from build123d import *

# Parameters (mm, degrees)
CROQUIS1_R              = 2.1
SALIENTE_EXTRUIR1_DEPTH = 7
CROQUIS2_R              = 2.1
CORTAR_EXTRUIR1_DEPTH   = 26.198920843
CORTAR_EXTRUIR2_DEPTH   = 26.198920843


with BuildPart() as part:
    # Croquis1 → Saliente-Extruir1 (new, symmetric)
    with BuildSketch(Plane(origin=(0, 0, 0), x_dir=(1, 0, 0), z_dir=(0, 1, 0))):
        with BuildLine():
            Line((0, 9.5), (-15, 9.5))
            Line((-15, 9.5), (-15, -9.499621356))
            Line((-15, -9.499621356), (0.084818048, -9.499621356))
            ThreePointArc((0.084818048, -9.499621356), (9.499905338, 0.042409446), (0, 9.5))
        make_face()
        with Locations(Location((0, 0, 0), (0, 0, 270))):
            Circle(CROQUIS1_R, mode=Mode.SUBTRACT)
    extrude(amount=SALIENTE_EXTRUIR1_DEPTH, both=True)

    # Croquis2 → Cortar-Extruir1 (cut, through all)
    with BuildSketch(Plane.XY.offset(9.499621356)):
        with Locations((-5, 0)):
            Circle(CROQUIS2_R)
    extrude(amount=-CORTAR_EXTRUIR1_DEPTH, mode=Mode.SUBTRACT)

    # Croquis3 → Cortar-Extruir2 (cut, through all)
    with BuildSketch(Plane.XY.offset(9.499621356)):
        with BuildLine():
            Line((-5, 7), (-15, 7))
            Line((-15, 7), (-15, -7))
            Line((-15, -7), (-5, -7))
            ThreePointArc((-5, -7), (-12, 0), (-5, 7))
        make_face()
    extrude(amount=-CORTAR_EXTRUIR2_DEPTH, mode=Mode.SUBTRACT)


solid = part.part
Read the model definition and answer for the solid it produces. Units are mm, in the model's axes. Give positions to 0.01 mm unless a question says otherwise; leave off trailing zeros. Write each loop counter-clockwise with the first axis right and the second up, starting at its lowest first coordinate (ties: lowest second). Pieces come first, ordered by that corner, then holes. Notation, with made-up numbers: (-8.5, 7.25) -> (44.5, 7.25) arc R23 ccw to (44.5, 19.25) -> close; hole circle Ø4 at (61, 29.5). An arc over 180 degrees is marked (long way). Answer as a JSON object with one key per item and string values. Group by question number.
1) Find section C-C (z = -5). Write down the section's boundary in (x, y), and give its area (3 significant figures).
2) Find section D-D (y = -2.75). Write down the section's boundary in (x, z).
3) Find section A-A (y = 0). Write down the section's boundary in (x, z).
4) The mould has two halves that part along X. Classify faces 1 (the cylindrical face through (-12, 0, 0)), 2 (the cylindrical face through (-2.997, 0.631, 0.133)), 3 (the flat face through (-7.25, 0.1, -9.5)), 4 (the cylindrical face through (0.631, -0.098, 2.003)): +X half, -X half, draft (parallel to the pull), parting line (faces both ways), or undercut.
5) Find section B-B (z = 0). Write down the section's boundary in (x, y), and give its area (3 significant figures).
6) Consider L1, parallel to Y at x = -5, z = -2.75; L2, parallel to Z at x = 1, y = 3; L3, parallel to Z at x = -1, y = 0. Determine where each line is inside the solid, lowest interval first. Write a range as from..to.
7) Each of these flat-tipped pins is pushed along its axis until it touches: P1, Ø5, axis at y = -1, z = -5.5, coming from the +X side; P2, Ø2, axis at x = 7, y = -5.5, coming from the +Z side; P3, Ø4, axis at x = -5, y = 0, coming from the -Z side. Where does it stop, or does it pass through?
Values follow:
{
 "1": {"outline": "(-5, -7) -> (8.08, -7) -> (8.08, 7) -> (-5, 7) arc R7 ccw to start; hole circle Ø4.2 at (-5, 0)", "area": "246 mm2"},
 "2": {"outline": "(-11.44, -9.5) -> (0, -9.5) arc R9.5 ccw to (0.08, 9.5) -> (-11.44, 9.5) -> close; hole circle Ø4.2 at (0, 0)"},
 "3": {"outline": "(-12, -9.5) -> (-7.1, -9.5) -> (-7.1, 9.5) -> (-12, 9.5) -> close; (-2.9, -9.5) -> (0, -9.5) arc R9.5 ccw to (0.08, 9.5) -> (-2.9, 9.5) -> close; hole circle Ø4.2 at (0, 0)"},
 "4": {"face 1": "-X half", "face 2": "undercut", "face 3": "draft", "face 4": "undercut"},
 "5": {"outline": "(-5, -7) -> (-2.1, -7) -> (-2.1, 7) -> (-5, 7) arc R7 ccw to start; (2.1, -7) -> (9.5, -7) -> (9.5, 7) -> (2.1, 7) -> close; hole circle Ø4.2 at (-5, 0)", "area": "207 mm2"},
 "6": {"L1": "y = -7..-2.1, 2.1..7", "L2": "z = -9.45..-1.85, 1.85..9.45", "L3": "z = -9.5..-1.85, 1.85..9.5"},
 "7": {"P1": "stops at x = 9.01", "P2": "stops at z = 7.37", "P3": "passes through"}
}
